```python
from build123d import *

# Parameters (mm, degrees)
F0_R     = 10
F1_DEPTH = 35
F2_R     = 5


# Not quite as in the source:
# - a feature names something its author has since deleted; it is built from what else it names


with BuildPart() as f1:
    # F0 (on Right) → F1 (new body)
    with BuildSketch(Plane.YZ):
        with BuildLine():
            Line((7.1040201683, -13.2110899417), (180.721386468, -5.3230686907))
            ThreePointArc((180.721386468, -5.3230686907), (220, 0), (180.721386468, 5.3230686907))
            Line((180.721386468, 5.3230686907), (7.1040201683, 13.2110899417))
            ThreePointArc((7.1040201683, 13.2110899417), (5.7575186768, 13.8510280733), (4.3541434669, 14.3541434669))
            Line((4.3541434669, 14.3541434669), (4.3541434669, 18.7082869339))
            Line((4.3541434669, 18.7082869339), (0, 18.7082869339))
            Line((0, 18.7082869339), (0, 14.3541434669))
            Line((0, 14.3541434669), (0, 10))
            ThreePointArc((0, 10), (10, 0), (0, -10))
            Line((0, -10), (0, -14.3541434669))
            Line((0, -14.3541434669), (0, -18.7082869339))
            Line((0, -18.7082869339), (4.3541434669, -18.7082869339))
            Line((4.3541434669, -18.7082869339), (4.3541434669, -14.3541434669))
            ThreePointArc((4.3541434669, -14.3541434669), (5.7575186768, -13.8510280733), (7.1040201683, -13.2110899417))
        make_face()
        with Locations((200, 0)):
            Circle(F0_R, mode=Mode.SUBTRACT)
    extrude(amount=F1_DEPTH)

    # F2
    f2_edges = [f1.edges().sort_by_distance(p)[0] for p in [
        (17.5, 7.10402, 13.21109),
        (17.5, 180.721386, 5.323069),
        (17.5, 180.721386, -5.323069),
        (17.5, 7.10402, -13.21109),
    ]]
    fillet(f2_edges, radius=F2_R)


solid = f1.part
```
For this review, take the finished solid that the model builds, in its own axes (mm). A direction names the side the tool comes from. Round coordinates to 2 decimals unless told otherwise and drop trailing zeros. Order: outer loops, then holes, each group sorted by start corner. A loop starts at its lowest first (then second) coordinate and runs counter-clockwise, first axis right, second up.
Q1. Wall thickness on line 1 (Z direction, x = 15.5, y = 200.5); line 2 (Y direction, x = 30, z = 3); line 3 (Y direction, x = 3.5, z = -15.5): over which ranges is each line inside the solid? List them lowest first.
Findings below:
line 1: z = -19.99 to -9.99, 9.99 to 19.99
line 2: y = 9.54 to 190.46, 209.54 to 219.77
line 3: y = 0 to 4.35, 187.36 to 212.64
Q2. We need section D-D, the plane y = 67.5. Give the boundary of the cut face in (x, z), plus the area to 3 significant figures.
Findings below:
outline: (0, -10.47) - (35, -10.47) - (35, 10.47) - (0, 10.47) - close
area: 733 mm2
Q3. Machinability: for faces 1 (the flat face through (35, 108, 0)), 2 (the flat face through (17, 4.354, -17)), 3 (the cylindrical face through (17.255, 219.986, -0.758)), 4 (the flat face through (17, 2, 18.708)), 5 (the flat face through (17, 4.354, 17)), which of the approach directions +Z, -Z, +X, -X, +Y, -Y give a long, thin tool a straight path to every point of the face, cutting with its end or side? Answer none if there is none.
Findings below:
face 1: +Z, -Z, +X, +Y, -Y
face 2: -Z, +X, -X
face 3: +X, -X
face 4: +Z, +X, -X, -Y
face 5: +Z, +X, -X
Q4. Mouldability with a two-part tool opening along Y and no side actions: class faces 6 (the flat face through (17.26, 91.43, -9.38)), 7 (the flat face through (17, 0, 14)), 8 (the flat face through (17, 2, -18.708)), 9 (the flat face through (17.255, 93.799, 9.272)) as pulls with the +Y half, pulls with the -Y half, needs draft (parallel to the pull), parting line crosses it, or undercut.
Findings below:
face 6: undercut
face 7: pulls with the -Y half
face 8: needs draft
face 9: undercut
Q5. We need section A-A, the plane z = 0. Give the boundary of the cut face in (x, y).
Findings below:
outline: (0, 10) - (35, 10) - (35, 190) - (0, 190) - close; (0, 210) - (35, 210) - (35, 220) - (0, 220) - close
Q6. We need section B-B, the plane x = 22. Give the boundary of the cut face in (y, z).
Findings below:
outline: (0, -18.71) - (4.35, -18.71) - (4.35, -14.35) arc R15 ccw to (6.29, -13.62) arc R5 cw to (8.16, -13.16) - (177.08, -5.49) arc R5 cw to (181.84, -8.39) arc R20 ccw (long way) to (181.84, 8.39) arc R5 cw to (177.08, 5.49) - (8.16, 13.16) arc R5 cw to (6.29, 13.62) arc R15 ccw to (4.35, 14.35) - (4.35, 18.71) - (0, 18.71) - (0, 10) arc R10 cw to (0, -10) - close; hole circle Ø20 at (200, 0)
Q7. We need section C-C, the plane y = 200. Give the boundary of the cut face in (x, z).
Findings below:
outline: (0, -20) - (35, -20) - (35, -10) - (0, -10) - close; (0, 10) - (35, 10) - (35, 20) - (0, 20) - close
Q8. Insertion check: P1, Ø1, axis at x = 22.5, z = 6, coming from the -Y side; P2, Ø12, axis at x = 14, y = 82.5, coming from the +Z side; P3, Ø2, axis at x = 23, y = 1.5, coming from the +Z side. Each pin has a flat end and moves straight along its axis. Give the tip position at first contact, or say it passes through.
Findings below:
P1: stops at y = 7.6
P2: stops at z = 10.06
P3: stops at z = 18.71
